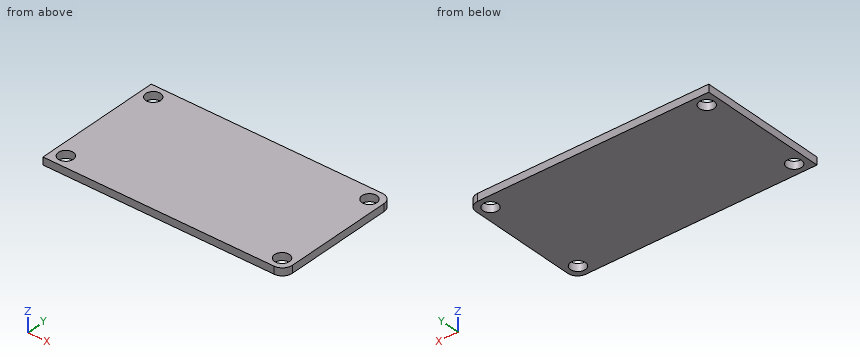
```python
from build123d import *

# Parameters (mm, degrees)
BOX_W        = 48.5
BOX_H        = 26
BOX_DEPTH    = 1.5
FILLET_R     = 2
SKETCH_R     = 1.5
POCKET_DEPTH = 5


with BuildPart() as part:
    # Box → Box (new body)
    with BuildSketch(Plane.XY):
        with Locations((24.25, 13)):
            Rectangle(BOX_W, BOX_H)
    extrude(amount=BOX_DEPTH)

    # Fillet
    fillet_edges = [part.edges().sort_by_distance(p)[0] for p in [
        (48.5, 0, 0.75),
        (48.5, 26, 0.75),
    ]]
    fillet(fillet_edges, radius=FILLET_R)

    # Sketch → Pocket (cut)
    with BuildSketch(Plane.XY.offset(1.5)):
        with Locations((2.5, 23.5)):
            Circle(SKETCH_R)
        with Locations((46, 23.5)):
            Circle(SKETCH_R)
        with Locations((46, 2.5)):
            Circle(SKETCH_R)
        with Locations((2.5, 2.5)):
            Circle(SKETCH_R)
    extrude(amount=-POCKET_DEPTH, mode=Mode.SUBTRACT)


solid = part.part
```
Here's how the part is built. I have some questions about the finished solid (model axes, mm). Coordinates: 2 decimals unless noted, no trailing zeros. Order: outer loops, then holes, each group sorted by start corner. A loop starts at its lowest first (then second) coordinate and runs counter-clockwise, first axis right, second up. Notation, with made-up numbers: (60, 47) - (119, 47) arc R29 ccw to (119, 78) - close; hole circle Ø1 at (-26, 51.5). An arc over 180 degrees is marked (long way). One line per question, with ' | ' between items.
(1) If I drill on L1, parallel to Y at x = 46, z = 0.35, over which ranges is the centre line in solid material (lowest first)?
Report:
L1: y = 0 to 1, 4 to 22, 25 to 26
(2) Suppose I cut it at C-C on y = 23.5. List the corners of the cut face in (x, z) for me, and give its area (4 significant figures).
Report:
outline: (0, 0) - (1, 0) - (1, 1.5) - (0, 1.5) - close; (4, 0) - (44.5, 0) - (44.5, 1.5) - (4, 1.5) - close; (47.5, 0) - (48.5, 0) - (48.5, 1.5) - (47.5, 1.5) - close | area: 63.75 mm2
(3) Suppose I cut it at B-B on z = 0.35. List the corners of the cut face in (x, y) for me.
Report:
outline: (0, 0) - (46.5, 0) arc R2 ccw to (48.5, 2) - (48.5, 24) arc R2 ccw to (46.5, 26) - (0, 26) - close; hole circle Ø3 at (2.5, 2.5); hole circle Ø3 at (2.5, 23.5); hole circle Ø3 at (46, 2.5); hole circle Ø3 at (46, 23.5)
(4) Suppose I cut it at A-A on x = 46. List the corners of the cut face in (y, z) for me, and give its area (3 significant figures).
Report:
outline: (0, 0) - (1, 0) - (1, 1.5) - (0, 1.5) - close; (4, 0) - (22, 0) - (22, 1.5) - (4, 1.5) - close; (25, 0) - (26, 0) - (26, 1.5) - (25, 1.5) - close | area: 30.0 mm2
